Geometry: final body of the model. Coordinates: model frame, mm. Face numbers are marked on the shaded views. Round coordinates to 2 decimals unless told otherwise and drop trailing zeros. Write each loop counter-clockwise with the first axis right and the second up, starting at its lowest first coordinate (ties: lowest second). Pieces come first, ordered by that corner, then holes. Notation, with made-up numbers: M 5.5,74 L 14.5,74 A8 ccw 14.5,84 Z; hole C 40.5,14.25 d4. An arc over 180 degrees is marked long. Use one line per item in the form item = value. Start each with the question number.
Item 1: Section query C-C (z = 21). Return loops of the section in (x, y), and give its area (3 significant figures).
Item 2: Ray query, probe 1 along Z at (x, y) = (0, -4.65); probe 2 along X at (y, z) = (-4.45, 15). Return the intervals inside material, ascending.
Item 3: Section query B-B (z = 5). Return loops of the section in (x, y), and give its area (3 significant figures).
Item 4: Pin query (flat end, axial travel): pin 1 Ø6 at (x, z) = (1.5, 7.5) entering from +Y; pin 2 Ø2 at (x, y) = (1.5, -2.5) entering from -Z; pin 3 Ø5 at (y, z) = (0, 5) entering from +X. Return the tip coordinate at first contact, or that it passes through.
Item 5: Section query D-D (x = -2.25). Return loops of the section in (y, z), and give its area (3 significant figures).
Item 6: Pull-direction query (Y, two-part tool) for the marked faces 1, 2 and 3; classes: pulls with the +Y half, pulls with the -Y half, needs draft (parallel to the pull), parting line crosses it, or undercut.
Item 7: Section query A-A (y = 0). Return loops of the section in (x, z).
from build123d import *

# Parameters (mm, degrees)
EXTRUDE_1_DEPTH          = 40
CUT_EXTRUDE_1_DEPTH      = 42.533119315
CUT_EXTRUDE_1_DEPTH_BACK = 42.533119315
SKETCH_2_R               = 1.6
SKETCH_3_R               = 1.6
CUT_EXTRUDE_2_DEPTH      = 42.533119315


with BuildPart() as part:
    # ｽｹｯﾁ1 → ﾎﾞｽ - 押し出し1 (new body)
    with BuildSketch(Plane.XY):
        Polygon((-4, 5), (-4, -4), (5, -4), (5, -5), (-5, -5), (-5, 5), align=None)
    extrude(amount=EXTRUDE_1_DEPTH)

    # ｽｹｯﾁ2 → ｶｯﾄ - 押し出し1 (cut, two sides: drawn at the far end of the back side and taken through both)
    with BuildSketch(Plane.XZ.offset(5).offset(-CUT_EXTRUDE_1_DEPTH_BACK)):
        with Locations(Location((0, 15, 0), (0, 0, 270))):
            Circle(SKETCH_2_R)
        with Locations(Location((0, 35, 0), (0, 0, 270))):
            Circle(SKETCH_2_R)
    extrude(amount=CUT_EXTRUDE_1_DEPTH + CUT_EXTRUDE_1_DEPTH_BACK, mode=Mode.SUBTRACT)

    # ｽｹｯﾁ3 → ｶｯﾄ - 押し出し2 (cut, through all)
    with BuildSketch(Plane.ZY.offset(5)):
        with Locations((5, 0)):
            Circle(SKETCH_3_R)
        with Locations((25, 0)):
            Circle(SKETCH_3_R)
    extrude(amount=-CUT_EXTRUDE_2_DEPTH, mode=Mode.SUBTRACT)


solid = part.part
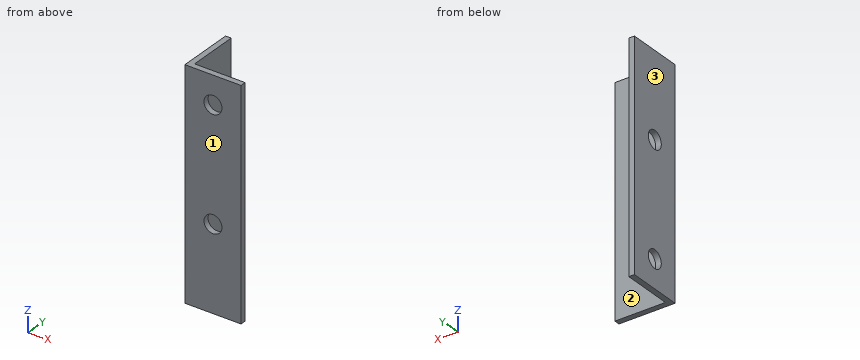
Working result:
q1.outline = M -5,-5 L 5,-5 L 5,-4 L -4,-4 L -4,5 L -5,5 Z
q1.area = 19.0 mm²
q2.probe_1 = 0 to 13.4, 16.6 to 33.4, 36.6 to 40
q2.probe_2 = -5 to -1.6, 1.6 to 5
q3.outline = M -5,-5 L 5,-5 L 5,-4 L -4,-4 L -4,-1.6 L -5,-1.6 Z; M -5,1.6 L -4,1.6 L -4,5 L -5,5 Z
q3.area = 15.8 mm²
q4.pin_1 = -4
q4.pin_2 = through
q4.pin_3 = -4
q5.outline = M -5,0 L -4,0 L -4,40 L -5,40 Z
q5.area = 40.0 mm²
q6.face_1 = pulls with the -Y half
q6.face_2 = pulls with the +Y half
q6.face_3 = needs draft
q7.outline = M -5,0 L -4,0 L -4,3.4 L -5,3.4 Z; M -5,6.6 L -4,6.6 L -4,23.4 L -5,23.4 Z; M -5,26.6 L -4,26.6 L -4,40 L -5,40 Z
